Can you work these out from the model? Positions are in its coordinate system, mm. Give positions to 0.01 mm unless a question says otherwise; leave off trailing zeros. Loops run counter-clockwise (first coordinate to the right, second up) from the corner with the lowest first, then second, coordinate; pieces in that order, holes last. Notation, with made-up numbers: (18, -31.75) - (37, -31.75) arc R29 ccw to (37, 5.25) - close; hole circle Ø10 at (-19.5, 59). An arc over 180 degrees is marked (long way). Answer as a JSON object with one key per item and string values. Group by question number.
Item 1: Suppose I cut it at B-B on x = 10. Write out the boundary of the cut face in (y, z), and give its area (3 significant figures).
Item 2: Suppose I cut it at C-C on x = 5.5. Write out the boundary of the cut face in (y, z).
Item 3: Suppose I cut it at D-D on y = -2.25. Write out the boundary of the cut face in (x, z).
Item 4: Suppose I cut it at A-A on z = 23.5. Write out the boundary of the cut face in (x, y).
Item 5: Please list where these lines run through material, in increasing order: L1, parallel to Y at x = 5.5, z = 26.5; L2, parallel to Z at x = 11.25, y = 4.5; L3, parallel to Z at x = -10.25, y = 1.25.
Item 6: Thinking about a two-plate mould opening in X: for faces 1 (the flat face through (0, 0, 40)), 2 (the flat face through (12.5, 0, 20)), 3 (the cylindrical face through (6.61, -1.99, 19.72)), 4 (the cylindrical face through (11.2, 0.1, 7.6)), which applies, pulls with the +X half, pulls with the -X half, needs draft (parallel to the pull), parting line crosses it, or undercut?
from build123d import *

# Parameters (mm, degrees)
F0_W     = 25
F0_H     = 12
F1_DEPTH = 40
F3_D     = 3
F5_D     = 3


# Not quite as in the source:
# - a feature names something its author has since deleted; it is built from what else it names


with BuildPart() as f1:
    # F0 (on Top) → F1 (new body)
    with BuildSketch(Plane.XY):
        Rectangle(F0_W, F0_H)
    extrude(amount=F1_DEPTH)

    # F3 (through all)
    with Locations(Plane.XZ.offset(6)):
        with Locations((-10, 23.5), (-10, 8.5), (10, 8.5), (10, 23.5)):
            Hole(F3_D / 2)

    # F5 (through all)
    with Locations(Plane.XY.offset(40)):
        with Locations((-5.5, -3), (5.5, -3), (-5.5, -3), (5.5, -3)):
            Hole(F5_D / 2)


solid = f1.part
Worked out:
{
 "1": {"outline": "(-6, 0) - (6, 0) - (6, 7) - (-6, 7) - close; (-6, 10) - (6, 10) - (6, 22) - (-6, 22) - close; (-6, 25) - (6, 25) - (6, 40) - (-6, 40) - close", "area": "408 mm2"},
 "2": {"outline": "(-6, 0) - (-4.5, 0) - (-4.5, 40) - (-6, 40) - close; (-1.5, 0) - (6, 0) - (6, 40) - (-1.5, 40) - close"},
 "3": {"outline": "(-12.5, 0) - (-6.8, 0) - (-6.8, 40) - (-12.5, 40) - close; (-4.2, 0) - (4.2, 0) - (4.2, 40) - (-4.2, 40) - close; (6.8, 0) - (12.5, 0) - (12.5, 40) - (6.8, 40) - close; hole circle Ø3 at (-10, 8.5); hole circle Ø3 at (-10, 23.5); hole circle Ø3 at (10, 8.5); hole circle Ø3 at (10, 23.5)"},
 "4": {"outline": "(-12.5, -6) - (-11.5, -6) - (-11.5, 6) - (-12.5, 6) - close; (-8.5, -6) - (8.5, -6) - (8.5, 6) - (-8.5, 6) - close; (11.5, -6) - (12.5, -6) - (12.5, 6) - (11.5, 6) - close; hole circle Ø3 at (-5.5, -3); hole circle Ø3 at (5.5, -3)"},
 "5": {"L1": "y = -6 to -4.5, -1.5 to 6", "L2": "z = 0 to 7.67, 9.33 to 22.67, 24.33 to 40", "L3": "z = 0 to 7.02, 9.98 to 22.02, 24.98 to 40"},
 "6": {"face 1": "needs draft", "face 2": "pulls with the +X half", "face 3": "undercut", "face 4": "undercut"}
}
